The model under review builds one solid part; all positions refer to its coordinate system, in mm. A direction names the side the tool comes from. Give positions to 0.01 mm unless a question says otherwise; leave off trailing zeros. Loops run counter-clockwise (first coordinate to the right, second up) from the corner with the lowest first, then second, coordinate; pieces in that order, holes last. Notation, with made-up numbers: M -38,28 L -31,28 A28 cw -31,65 Z; hole C 2,58 d5. An arc over 180 degrees is marked long. One line per item, written item: value. Start each with the question number.
Q1. We need section A-A on x = 0. Write out the cut boundary in (y, z) (3 decimals).
Q2. For pin 1 (2 mm diameter, centred on y = 9.5, z = -4, fed in from -X); pin 2 (4 mm diameter, centred on x = -6, y = 6.5, fed in from -Z); pin 3 (1.3 mm diameter, centred on x = 0.5, z = 7.5, fed in from +Y), all flat-tipped, find the tip position at first contact; note any pin that passes through.
Q3. To check wall thickness, follow line 1 along X through (y, z) = (4, -0.5); line 2 along Z through (x, y) = (-0.75, 7.25); line 3 along X through (y, z) = (11, -1). State the ranges of each line that lie inside material, in increasing order. Write a range as from..to.
Q4. We need section B-B on z = 0. Write out the cut boundary in (x, y) (3 decimals), plus the area to 4 significant figures.
Q5. We need section D-D on y = 10. Write out the cut boundary in (x, z).
Q6. For faces 1 (the face through (-0.045, 3.296, -8.524)), 2 (the face through (6.212, 9.796, 0.406)), list the 3-axis set-ups (+Z, -Z, +X, -X, +Y, -Y) from which the entire face can be reached by the end or side of a thin tool; tool diameter is ignored.
Q7. We need section C-C on z = 7.5. Write out the cut boundary in (x, y) (3 decimals).
Q8. Mouldability with a two-part tool opening along Z and no side actions: class faces 3 (the face through (9.76, 6.41, 2.17)), 4 (the face through (-5, 13, -2)), 5 (the face through (0.406, 9.796, -6.212)) as released by +Z, released by -Z, zero draft, split by the parting line, or undercut.
```python
from build123d import *

# Parameters (mm, degrees)
SKETCH_1_R               = 10
SKETCH_1_R_2             = 5
EXTRUDE_1_DEPTH          = 13
SKETCH_2_R               = 1.35
CUT_EXTRUDE_1_DEPTH      = 6.5
PATTERN_CIRCULAR_1_COUNT = 4


with BuildPart() as part:
    # 草图1 → 凸台-拉伸1 (new body)
    with BuildSketch(Plane(origin=(0, 0, 0), x_dir=(1, 0, 0), z_dir=(0, 1, 0))):
        with Locations(Location((0, 0, 0), (0, 0, 90))):
            Circle(SKETCH_1_R)
        with Locations(Location((0, 0, 0), (0, 0, 90))):
            Circle(SKETCH_1_R_2, mode=Mode.SUBTRACT)
    extrude(amount=EXTRUDE_1_DEPTH)

    # 草图2 → 切除-拉伸1 (cut)
    with BuildSketch(Plane(origin=(0, 13, 0), x_dir=(1, 0, 0), z_dir=(0, 1, 0))):
        with Locations(Location((0, 7.5, 0), (0, 0, 270))):
            Circle(SKETCH_2_R)
    cut_extrude_1 = extrude(amount=-CUT_EXTRUDE_1_DEPTH, mode=Mode.SUBTRACT)

    # 草图5 → M2.5 螺纹孔1 (revolve, cut)
    with BuildSketch(Plane(origin=(0, 6.5, -7.5), x_dir=(0, 0, 1), z_dir=(1, 0, 0))):
        Polygon((0, 0), (0, 27.865882135), (1.025, 27.25), (1.025, 0), align=None)
    hole_wizard_m2_5_1 = revolve(axis=Axis((0, 12.85, -7.5), (0, -1, 0)), mode=Mode.SUBTRACT)

    # 阵列(圆周)1: 切除-拉伸1, M2.5 螺纹孔1 ×4 about axis
    pattern_circular_1_axis = Axis((0, 0, 0), (0, 1, 0))
    add([cut_extrude_1.rotate(pattern_circular_1_axis, i * 360 / PATTERN_CIRCULAR_1_COUNT) for i in range(1, PATTERN_CIRCULAR_1_COUNT)], mode=Mode.SUBTRACT)
    add([hole_wizard_m2_5_1.rotate(pattern_circular_1_axis, i * 360 / PATTERN_CIRCULAR_1_COUNT) for i in range(1, PATTERN_CIRCULAR_1_COUNT)], mode=Mode.SUBTRACT)


solid = part.part
```
Solved:
1. outline: M 0,-10 L 13,-10 L 13,-8.85 L 6.5,-8.85 L 6.5,-8.525 L 0,-8.525 Z; M 0,-6.475 L 6.5,-6.475 L 6.5,-6.15 L 13,-6.15 L 13,-5 L 0,-5 Z; M 0,5 L 13,5 L 13,6.15 L 6.5,6.15 L 6.5,6.475 L 0,6.475 Z; M 0,8.525 L 6.5,8.525 L 6.5,8.85 L 13,8.85 L 13,10 L 0,10 Z
2. pin 1: x = -9.54
2. pin 2: z = -9.17
2. pin 3: y = 6.5
3. line 1: -9.99..-8.39, -6.61..-4.97, 4.97..6.61, 8.39..9.99
3. line 2: -9.97..-8.62, -6.38..-4.94, 4.94..6.38, 8.62..9.97
3. line 3: -9.95..-8.41, -6.59..-4.9, 4.9..6.59, 8.41..9.95
4. outline: M -10,0 L -8.525,0 L -8.525,6.5 L -8.85,6.5 L -8.85,13 L -10,13 Z; M -6.475,0 L -5,0 L -5,13 L -6.15,13 L -6.15,6.5 L -6.475,6.5 Z; M 5,0 L 6.475,0 L 6.475,6.5 L 6.15,6.5 L 6.15,13 L 5,13 Z; M 8.525,0 L 10,0 L 10,13 L 8.85,13 L 8.85,6.5 L 8.525,6.5 Z
4. area: 68.25 mm2
5. outline: C 0,0 d20; hole C -7.5,0 d2.7; hole C 0,0 d10; hole C 0,-7.5 d2.7; hole C 0,7.5 d2.7; hole C 7.5,0 d2.7
6. face 1: +Y, -Y
6. face 2: +Y
7. outline: M -6.614,0 L -1.025,0 L -1.025,6.5 L -1.35,6.5 L -1.35,13 L -6.614,13 Z; M 1.025,0 L 6.614,0 L 6.614,13 L 1.35,13 L 1.35,6.5 L 1.025,6.5 Z
8. face 3: split by the parting line
8. face 4: zero draft
8. face 5: undercut
